from build123d import *

# Parameters (mm, degrees)
BASE_W                   = 220
BASE_H                   = 420
BASE_W_2                 = 380
PLANCHE_BAS_DEPTH        = 10
BASE_6_W                 = 10
BASE_6_H                 = 420
PANNEAUX_LATERAUX_DEPTH  = 580
BASE_7_W                 = 10
BASE_7_H                 = 420
PANNEAUX_BAS_INTER_DEPTH = 390
ESQUISSE2_W              = 380
ESQUISSE2_H              = 420
BOSS_EXTRU_9_DEPTH       = 10
ESQUISSE2_W_2            = 440
BOSS_EXTRU_9_2_DEPTH     = 10
ESQUISSE2_W_3            = 280
ESQUISSE2_H_2            = 20
BOSS_EXTRU_9_3_DEPTH     = 10
ESQUISSE2_4_W            = 10
ESQUISSE2_4_H            = 420
BOSS_EXTRU_10_DEPTH      = 190
ESQUISSE5_W              = 1240
ESQUISSE5_H              = 420
ESQUISSE5_W_2            = 330
ESQUISSE5_H_2            = 290
ESQUISSE5_W_3            = 440
ESQUISSE5_H_3            = 380
BOSS_EXTRU_11_DEPTH      = 10
ESQUISSE7_W              = 440
ESQUISSE7_H              = 380
BOSS_EXTRU_12_DEPTH      = 10
BOSS_EXTRU_13_DEPTH      = 30
BOSS_EXTRU_13_DEPTH_BACK = 10
ESQUISSE7_3_W            = 440
ESQUISSE7_3_H            = 20
ESQUISSE8_W              = 330
ESQUISSE8_H              = 135
ENL_V_MAT_EXTRU_3_DEPTH  = 10
ESQUISSE2_5_W            = 280
ESQUISSE2_5_H            = 20
BOSS_EXTRU_14_DEPTH      = 20


with BuildPart() as part:
    # base → planche_bas (new body)
    with BuildSketch(Plane(origin=(0, 0, 0), x_dir=(1, 0, 0), z_dir=(0, 1, 0))):
        with Locations((106.826222685, -21.477627471)):
            Rectangle(BASE_W, BASE_H)
        with Locations((-113.173777315, -21.477627471)):
            Rectangle(BASE_W, BASE_H)
        with Locations((416.826222685, -21.477627471)):
            Rectangle(BASE_W_2, BASE_H)
        with Locations((-423.173777315, -21.477627471)):
            Rectangle(BASE_W_2, BASE_H)
    extrude(amount=PLANCHE_BAS_DEPTH)

    # base_6 → panneaux_lateraux (add)
    with BuildSketch(Plane(origin=(0, 0, 0), x_dir=(1, 0, 0), z_dir=(0, 1, 0))):
        with Locations((611.826222685, -21.477627471)):
            Rectangle(BASE_6_W, BASE_6_H)
        with Locations((-618.173777315, -21.477627471)):
            Rectangle(BASE_6_W, BASE_6_H)
    extrude(amount=PANNEAUX_LATERAUX_DEPTH)

    # base_7 → panneaux_bas_inter (add)
    with BuildSketch(Plane(origin=(0, 0, 0), x_dir=(1, 0, 0), z_dir=(0, 1, 0))):
        with Locations((221.826222685, -21.477627471)):
            Rectangle(BASE_7_W, BASE_7_H)
        with Locations((-228.173777315, -21.477627471)):
            Rectangle(BASE_7_W, BASE_7_H)
    extrude(amount=PANNEAUX_BAS_INTER_DEPTH)



with BuildPart() as body_2:
    # Esquisse2 → Boss.-Extru.9 (new body)
    with BuildSketch(Plane(origin=(0, 390, 0), x_dir=(1, 0, 0), z_dir=(0, 1, 0))):
        with Locations((-423.173777315, -21.477627471)):
            Rectangle(ESQUISSE2_W, ESQUISSE2_H)
    extrude(amount=BOSS_EXTRU_9_DEPTH)


with BuildPart() as body_3:
    # Esquisse2 → Boss.-Extru.9 2 (new body)
    with BuildSketch(Plane(origin=(0, 390, 0), x_dir=(1, 0, 0), z_dir=(0, 1, 0))):
        with Locations((-3.173777315, -21.477627471)):
            Rectangle(ESQUISSE2_W_2, ESQUISSE2_H)
    extrude(amount=BOSS_EXTRU_9_2_DEPTH)


with BuildPart() as body_4:
    # Esquisse2 → Boss.-Extru.9 3 (new body)
    with BuildSketch(Plane(origin=(0, 390, 0), x_dir=(1, 0, 0), z_dir=(0, 1, 0))):
        with Locations((416.826222685, -21.477627471)):
            Rectangle(ESQUISSE2_W, ESQUISSE2_H)
        with Locations((416.826222685, -201.477627471)):
            Rectangle(ESQUISSE2_W_3, ESQUISSE2_H_2, mode=Mode.SUBTRACT)
    extrude(amount=BOSS_EXTRU_9_3_DEPTH)


with BuildPart() as part_1:
    add(part.part)

    add(body_2.part)  # Boss.-Extru.10 merges body 2

    add(body_3.part)  # Boss.-Extru.10 merges body 3

    add(body_4.part)  # Boss.-Extru.10 merges body 4
    # Esquisse2_4 → Boss.-Extru.10 (add)
    with BuildSketch(Plane(origin=(0, 390, 0), x_dir=(1, 0, 0), z_dir=(0, 1, 0))):
        with Locations((-228.173777315, -21.477627471)):
            Rectangle(ESQUISSE2_4_W, ESQUISSE2_4_H)
        with Locations((221.826222685, -21.477627471)):
            Rectangle(ESQUISSE2_4_W, ESQUISSE2_4_H)
    extrude(amount=BOSS_EXTRU_10_DEPTH)

    # Esquisse5 → Boss.-Extru.11 (add)
    with BuildSketch(Plane(origin=(0, 580, 0), x_dir=(1, 0, 0), z_dir=(0, 1, 0))):
        with Locations((-3.173777315, -21.477627471)):
            Rectangle(ESQUISSE5_W, ESQUISSE5_H)
        with Locations((416.826222685, -21.477627471)):
            Rectangle(ESQUISSE5_W_2, ESQUISSE5_H_2, mode=Mode.SUBTRACT)
        with Locations((-3.173777315, -21.477627471)):
            Rectangle(ESQUISSE5_W_3, ESQUISSE5_H_3, mode=Mode.SUBTRACT)
    extrude(amount=BOSS_EXTRU_11_DEPTH)

    # Esquisse7 → Boss.-Extru.12 (add)
    with BuildSketch(Plane(origin=(0, 550, 0), x_dir=(1, 0, 0), z_dir=(0, 1, 0))):
        with Locations((-3.173777315, -21.477627471)):
            Rectangle(ESQUISSE7_W, ESQUISSE7_H)
    extrude(amount=-BOSS_EXTRU_12_DEPTH)

    # Esquisse7_3 → Boss.-Extru.13 (add, two sides: drawn at the far end of the back side and taken through both)
    with BuildSketch(Plane(origin=(0, 550, 0), x_dir=(1, 0, 0), z_dir=(0, 1, 0)).offset(-BOSS_EXTRU_13_DEPTH_BACK)):
        with Locations((-3.173777315, -221.477627471)):
            Rectangle(ESQUISSE7_3_W, ESQUISSE7_3_H)
    extrude(amount=BOSS_EXTRU_13_DEPTH + BOSS_EXTRU_13_DEPTH_BACK)

    # Esquisse8 → Enl_v. mat.-Extru.3 (cut)
    with BuildSketch(Plane(origin=(616.826222685, 0, 0), x_dir=(0, 0, -1), z_dir=(1, 0, 0))):
        with Locations((-21.477627471, 477.5)):
            Rectangle(ESQUISSE8_W, ESQUISSE8_H)
    extrude(amount=-ENL_V_MAT_EXTRU_3_DEPTH, mode=Mode.SUBTRACT)

    # Esquisse2_5 → Boss.-Extru.14 (add)
    with BuildSketch(Plane(origin=(0, 390, 0), x_dir=(1, 0, 0), z_dir=(0, 1, 0))):
        with Locations((416.826222685, -201.477627471)):
            Rectangle(ESQUISSE2_5_W, ESQUISSE2_5_H)
    extrude(amount=BOSS_EXTRU_14_DEPTH)


solid = part_1.part
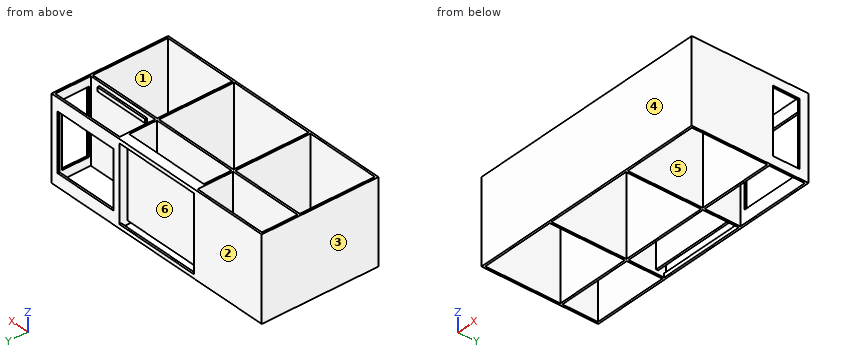
For this review, take the finished solid that the model builds, in its own axes (mm). Face numbers are marked on the shaded views. A direction names the side the tool comes from. Round coordinates to 2 decimals unless told otherwise and drop trailing zeros. Loops run counter-clockwise (first coordinate to the right, second up) from the corner with the lowest first, then second, coordinate; pieces in that order, holes last. Notation, with made-up numbers: (25, 71.25) - (83, 71.25) arc R21 ccw to (83, 97.25) - close; hole circle Ø9 at (57, 15). An arc over 180 degrees is marked (long way). One line per item, written item: value. Start each with the question number.
Item 1: Take a section at A-A (x = 442). Give the boundary of the cut face in (y, z), plus the area to 3 significant figures.
Item 2: For the marked faces 4, 5 and 6, list the 3-axis set-ups (+Z, -Z, +X, -X, +Y, -Y) from which the entire face can be reached by the end or side of a thin tool; tool diameter is ignored.
Item 3: Take a section at C-C (z = 91). State how many separate pieces and enclosed holes the cut face has, plus the area to 4 significant figures.
Item 4: Take a section at B-B (y = 48). Give the boundary of the cut face in (x, z), plus the area to 3 significant figures.
Item 5: Clearance check with flat-ended pins moving along their axes: pin 1 Ø2 at (x, z) = (-3, -53.5) entering from +Y; pin 2 Ø3 at (x, y) = (424, 403) entering from +Z; pin 3 Ø8 at (x, y) = (66, 547) entering from -Z. State where each tip first meets the part, or that it passes through.
Item 6: For L1, parallel to Y at x = -285.5, z = -32.5; L2, parallel to X at y = 387, z = -76.5; L3, parallel to X at y = 524, z = 7, list the stretches that pass through material, from the lowest coordinate up.
Item 7: The part is to be moulded in two halves that separate along Y. For the marked faces 1, 2 and 3, say which applies: +Y half, -Y half, draft (parallel to the pull), parting line (faces both ways), or undercut.
Item 8: Take a section at D-D (y = 496). Give the boundary of the cut face in (x, z).
Answer below:
1. outline: (0, -188.52) - (10, -188.52) - (10, 231.48) - (0, 231.48) - close; (390, -188.52) - (400, -188.52) - (400, 191.48) - (410, 191.48) - (410, 211.48) - (400, 211.48) - (400, 231.48) - (390, 231.48) - close; (580, -188.52) - (590, -188.52) - (590, -123.52) - (580, -123.52) - close; (580, 166.48) - (590, 166.48) - (590, 231.48) - (580, 231.48) - close
1. area: 9,900 mm2
2. face 4: +Z, -Z, +X, -X, -Y
2. face 5: +Z, -Z
2. face 6: -Z, +Y
3. separate pieces: 2
3. enclosed holes: 5
3. area: 54,950 mm2
4. outline: (-623.17, -188.52) - (-613.17, -188.52) - (-613.17, 231.48) - (-623.17, 231.48) - close; (-233.17, -188.52) - (-223.17, -188.52) - (-223.17, 231.48) - (-233.17, 231.48) - close; (216.83, -188.52) - (226.83, -188.52) - (226.83, 231.48) - (216.83, 231.48) - close; (606.83, -188.52) - (616.83, -188.52) - (616.83, 231.48) - (606.83, 231.48) - close
4. area: 16,800 mm2
5. pin 1: stops at y = 550
5. pin 2: stops at z = 211.48
5. pin 3: stops at z = -168.52
6. L1: y = 0 to 10, 390 to 400, 580 to 590
6. L2: x = -623.17 to -613.17, -233.17 to -223.17, 216.83 to 226.83, 606.83 to 616.83
6. L3: x = -623.17 to -613.17, -233.17 to -223.17, 216.83 to 226.83
7. face 1: undercut
7. face 2: +Y half
7. face 3: draft
8. outline: (-623.17, -188.52) - (-613.17, -188.52) - (-613.17, 231.48) - (-623.17, 231.48) - close; (-233.17, -188.52) - (-223.17, -188.52) - (-223.17, 231.48) - (-233.17, 231.48) - close; (216.83, -188.52) - (226.83, -188.52) - (226.83, 231.48) - (216.83, 231.48) - close; (606.83, -188.52) - (616.83, -188.52) - (616.83, -143.52) - (606.83, -143.52) - close; (606.83, 186.48) - (616.83, 186.48) - (616.83, 231.48) - (606.83, 231.48) - close
